```python
from build123d import *

# Parameters (mm, degrees)
F0_W     = 22.854749
F0_H     = 98.96972
F1_DEPTH = 25.4
F3_DEPTH = 22.855749
F4_DEPTH = 50.8
F6_DEPTH = 22.855749


with BuildPart() as f1:
    # F0 (on Right) → F1 (new body)
    with BuildSketch(Plane.YZ):
        with Locations((-34.282123, 0)):
            Rectangle(F0_W, F0_H)
    extrude(amount=F1_DEPTH)

    # F2 (on face) → F3 (cut, through all)
    with BuildSketch(Plane.XZ.offset(45.709498)):
        Polygon((25.4, 49.48486), (12.7, 49.48486), (25.4, -49.48486), align=None)
    extrude(amount=-F3_DEPTH, mode=Mode.SUBTRACT)

    # F0 (on Right) → F4 (join)
    with BuildSketch(Plane.YZ):
        Polygon((0, -49.48486), (0, 0), (0, 49.48486), (-22.854749, 49.48486), (-22.854749, -49.48486), align=None)
    extrude(amount=F4_DEPTH)

    # F5 (on face) → F6 (cut, through all)
    with BuildSketch(Plane.XZ.offset(22.854749)):
        Polygon((50.8, 49.48486), (31.75, 49.48486), (50.8, -49.48486), align=None)
    extrude(amount=-F6_DEPTH, mode=Mode.SUBTRACT)

    # F7: F1 across plane


with BuildPart() as f1_1:
    add(f1.part)
    add(f1.part.mirror(Plane.XZ))


solid = f1_1.part
```
Could you check a few things on this model? Use its own coordinates, in mm. A direction names the side the tool comes from. Round coordinates to 2 decimals unless told otherwise and drop trailing zeros. Loops run counter-clockwise (first coordinate to the right, second up) from the corner with the lowest first, then second, coordinate; pieces in that order, holes last.
Q1. I want a section at D-D (x = 27). Write out the boundary of the cut face in (y, z), and give its area (3 significant figures).
Q2. I want a section at C-C (y = 12.5). Write out the boundary of the cut face in (x, z).
Q3. I want a section at A-A (z = -42). Write out the boundary of the cut face in (x, y).
Q4. I want a section at B-B (x = 15). Write out the boundary of the cut face in (y, z).
Q5. For P1, Ø2, axis at x = 42.5, z = -36, coming from the +Y side; P2, Ø2, axis at y = -3.5, z = 28, coming from the +X side; P3, Ø4, axis at y = 7.5, z = -3, coming from the +X side, each with a flat end and sliding along its axis, tell me the tip position at first contact or that it passes through.
Q6. On a 3-axis mill with a long thin cutter (end or side, diameter ignored), from which of +Z, -Z, +X, -X, +Y, -Y can I reach the whole of each face in a straight line? I mean faces 1 (the flat face through (31, -22.855, 1)), 2 (the flat face through (18.96, 34.44, 0.69)), 3 (the flat face through (19, 1, -49.485)). Say none if no direction works.
Q7. Please list where these lines run through material, in increasing order: L1, parallel to Y at x = 34, z = -31; L2, parallel to X at y = -37, z = 4.5; L3, parallel to X at y = 32, z = -17.5.
Answer below:
1. outline: (-22.85, -49.48) - (22.85, -49.48) - (22.85, 49.48) - (-22.85, 49.48) - close
1. area: 4,520 mm2
2. outline: (0, -49.48) - (50.8, -49.48) - (31.75, 49.48) - (0, 49.48) - close
3. outline: (0, -45.71) - (24.44, -45.71) - (24.44, -22.85) - (49.36, -22.85) - (49.36, 22.85) - (24.44, 22.85) - (24.44, 45.71) - (0, 45.71) - close
4. outline: (-45.71, -49.48) - (45.71, -49.48) - (45.71, 31.56) - (22.85, 31.56) - (22.85, 49.48) - (-22.85, 49.48) - (-22.85, 31.56) - (-45.71, 31.56) - close
5. P1: stops at y = 22.85
5. P2: stops at x = 36.08
5. P3: stops at x = 42.24
6. face 1: +Z, +X, -Y
6. face 2: +Z, +X, +Y
6. face 3: -Z, +X, -X, +Y, -Y
7. L1: y = -22.85 to 22.85
7. L2: x = 0 to 18.47
7. L3: x = 0 to 21.3
